from build123d import *

# Parameters (mm, degrees)
CROQUIS1_R              = 7.5
CROQUIS1_R_2            = 5
SALIENTE_EXTRUIR1_DEPTH = 2
CHAFL_N1_SIZE           = 0.5
CROQUIS2_R              = 6.611271869
CROQUIS2_R_2            = 5.520857639
SALIENTE_EXTRUIR2_DEPTH = 2.05


with BuildPart() as part:
    # Croquis1 → Saliente-Extruir1 (new, symmetric)
    with BuildSketch(Plane(origin=(0, 0, 0), x_dir=(1, 0, 0), z_dir=(0, 1, 0))):
        with Locations(Location((0, 0, 0), (0, 0, 270))):
            Circle(CROQUIS1_R)
        with Locations(Location((0, 0, 0), (0, 0, 270))):
            Circle(CROQUIS1_R_2, mode=Mode.SUBTRACT)
    extrude(amount=SALIENTE_EXTRUIR1_DEPTH, both=True)

    # Chaflán1
    chafl_n1_edges = [part.edges().sort_by_distance(p)[0] for p in [
        (0, -2, -7.5),
        (0, 2, -7.5),
    ]]
    chamfer(chafl_n1_edges, length=CHAFL_N1_SIZE)

    # Croquis2 → Saliente-Extruir2 (add, symmetric)
    with BuildSketch(Plane(origin=(0, 0, 0), x_dir=(1, 0, 0), z_dir=(0, 1, 0))):
        with Locations(Location((0, 0, 0), (0, 0, 270))):
            Circle(CROQUIS2_R)
        with Locations(Location((0, 0, 0), (0, 0, 270))):
            Circle(CROQUIS2_R_2, mode=Mode.SUBTRACT)
    extrude(amount=SALIENTE_EXTRUIR2_DEPTH, both=True)


solid = part.part
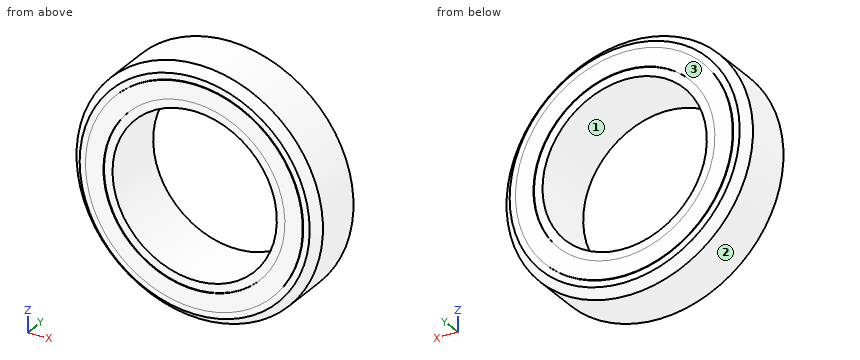
Part model, mm, in its own coordinate system. Face numbers are marked on the shaded views. Coordinates: 2 decimals unless noted, no trailing zeros. Write each loop counter-clockwise with the first axis right and the second up, starting at its lowest first coordinate (ties: lowest second). Pieces come first, ordered by that corner, then holes. Notation, with made-up numbers: (48, 22.5) - (104, 22.5) arc R21 cw to (104, 39.5) - close; hole circle Ø8 at (66, -24). An arc over 180 degrees is marked (long way). Put each result on its own line as item: value.
1. Flat gauge pins, fed straight in: pin 1 Ø1.5 at (y, z) = (-1.5, 3.5) entering from -X; pin 2 Ø1.5 at (y, z) = (-1.5, 5.5) entering from +X; pin 3 Ø5.5 at (x, z) = (1.5, 0) entering from -Y; pin 4 Ø1.5 at (y, z) = (0.5, 1) entering from -X. Where does each tip first touch, or does it go through?
Final values:
pin 1: stops at x = -6.98
pin 2: stops at x = 5.8
pin 3: passes through
pin 4: stops at x = -7.5
2. Band-saw the part on C-C (y = 0.8). Write the cut outline in (x, z).
Final values:
outline: circle Ø15 at (0, 0); hole circle Ø10 at (0, 0)
3. Band-saw the part on A-A (z = 0). Write the cut outline in (x, y).
Final values:
outline: (-7.5, -1.5) - (-7, -2) - (-6.61, -2) - (-6.61, -2.05) - (-5.52, -2.05) - (-5.52, -2) - (-5, -2) - (-5, 2) - (-5.52, 2) - (-5.52, 2.05) - (-6.61, 2.05) - (-6.61, 2) - (-7, 2) - (-7.5, 1.5) - close; (5, -2) - (5.52, -2) - (5.52, -2.05) - (6.61, -2.05) - (6.61, -2) - (7, -2) - (7.5, -1.5) - (7.5, 1.5) - (7, 2) - (6.61, 2) - (6.61, 2.05) - (5.52, 2.05) - (5.52, 2) - (5, 2) - close
4. Band-saw the part on B-B (x = 0). Write the cut outline in (y, z).
Final values:
outline: (-2.05, -6.61) - (-2, -6.61) - (-2, -7) - (-1.5, -7.5) - (1.5, -7.5) - (2, -7) - (2, -6.61) - (2.05, -6.61) - (2.05, -5.52) - (2, -5.52) - (2, -5) - (-2, -5) - (-2, -5.52) - (-2.05, -5.52) - close; (-2.05, 5.52) - (-2, 5.52) - (-2, 5) - (2, 5) - (2, 5.52) - (2.05, 5.52) - (2.05, 6.61) - (2, 6.61) - (2, 7) - (1.5, 7.5) - (-1.5, 7.5) - (-2, 7) - (-2, 6.61) - (-2.05, 6.61) - close
5. Two-plate mould, pull along Z, no slides. Class the marked faces 1, 2 and 3: +Z half, -Z half, draft (parallel to the pull), parting line (faces both ways), or undercut.
Final values:
face 1: undercut
face 2: parting line
face 3: draft
6. Probe line 1 along X through (y, z) = (-0.9, 0); line 2 along X through (y, z) = (1.8, 0.25); line 3 along Z through (x, y) = (0.25, 1). List the from-to ranges inside material, lowest first. Write a range as [from, to].
Final values:
line 1: x = [-7.5, -5], [5, 7.5]
line 2: x = [-7.2, -4.99], [4.99, 7.2]
line 3: z = [-7.5, -4.99], [4.99, 7.5]
